from build123d import *

# Parameters (mm, degrees)
F3_DEPTH = 50
F4_DEPTH = 50
F5_DEPTH = 50


with BuildPart() as f3:
    # F0 (on Top) → F3 (new body, symmetric)
    with BuildSketch(Plane.XY):
        with BuildLine():
            Line((-30, 30), (45, 30))
            ThreePointArc((45, 30), (48.535534, 31.464466), (50, 35))
            Line((50, 35), (50, 45))
            ThreePointArc((50, 45), (48.535534, 48.535534), (45, 50))
            Line((45, 50), (-45, 50))
            ThreePointArc((-45, 50), (-48.535534, 48.535534), (-50, 45))
            Line((-50, 45), (-50, -45))
            ThreePointArc((-50, -45), (-48.535534, -48.535534), (-45, -50))
            Line((-45, -50), (45, -50))
            ThreePointArc((45, -50), (48.535534, -48.535534), (50, -45))
            Line((50, -45), (50, 4.584678))
            ThreePointArc((50, 4.584678), (48.535534, 8.120212), (45, 9.584678))
            Line((45, 9.584678), (-16.822587, 9.584678))
            ThreePointArc((-16.822587, 9.584678), (-20.358121, 8.120212), (-21.822587, 4.584678))
            Line((-21.822587, 4.584678), (-21.822587, -15.415322))
            ThreePointArc((-21.822587, -15.415322), (-20.358121, -18.950856), (-16.822587, -20.415322))
            Line((-16.822587, -20.415322), (-13.330647, -20.415322))
            ThreePointArc((-13.330647, -20.415322), (-9.795113, -18.950856), (-8.330647, -15.415322))
            Line((-8.330647, -15.415322), (-8.330647, -5.415322))
            Line((-8.330647, -5.415322), (30, -5.415322))
            Line((30, -5.415322), (30, -30))
            Line((30, -30), (-30, -30))
            Line((-30, -30), (-30, 30))
        make_face()
    extrude(amount=F3_DEPTH, both=True)

    # F1 (on Front) → F4 (intersect, symmetric)
    with BuildSketch(Plane.XZ):
        with BuildLine():
            Line((-33.193547, 7.949598), (-33.193547, 31.362906))
            Line((-33.193547, 31.362906), (45, 31.362906))
            ThreePointArc((45, 31.362906), (48.535534, 32.827372), (50, 36.362906))
            Line((50, 36.362906), (50, 45))
            ThreePointArc((50, 45), (48.535534, 48.535534), (45, 50))
            Line((45, 50), (-45, 50))
            ThreePointArc((-45, 50), (-48.535534, 48.535534), (-50, 45))
            Line((-50, 45), (-50, -45))
            ThreePointArc((-50, -45), (-48.535534, -48.535534), (-45, -50))
            Line((-45, -50), (45, -50))
            ThreePointArc((45, -50), (48.535534, -48.535534), (50, -45))
            Line((50, -45), (50, -37.162689))
            ThreePointArc((50, -37.162689), (48.535534, -33.627155), (45, -32.162689))
            Line((45, -32.162689), (-31.415325, -32.162689))
            Line((-31.415325, -32.162689), (-31.415325, -9.536289))
            Line((-31.415325, -9.536289), (45, -9.536289))
            ThreePointArc((45, -9.536289), (48.535534, -8.071823), (50, -4.536289))
            Line((50, -4.536289), (50, 2.949598))
            ThreePointArc((50, 2.949598), (48.535534, 6.485132), (45, 7.949598))
            Line((45, 7.949598), (-33.193547, 7.949598))
        make_face()
    extrude(amount=F4_DEPTH, both=True, mode=Mode.INTERSECT)

    # F2 (on Right) → F5 (intersect, symmetric)
    with BuildSketch(Plane.YZ):
        with BuildLine():
            ThreePointArc((-45, 50), (-48.535534, 48.535534), (-50, 45))
            Line((-50, 45), (-50, -5))
            ThreePointArc((-50, -5), (-48.535534, -8.535534), (-45, -10))
            Line((-45, -10), (30, -10))
            Line((30, -10), (30, -30))
            Line((30, -30), (-45, -30))
            ThreePointArc((-45, -30), (-48.535534, -31.464466), (-50, -35))
            Line((-50, -35), (-50, -45))
            ThreePointArc((-50, -45), (-48.535534, -48.535534), (-45, -50))
            Line((-45, -50), (45, -50))
            ThreePointArc((45, -50), (48.535534, -48.535534), (50, -45))
            Line((50, -45), (50, 5))
            ThreePointArc((50, 5), (48.535534, 8.535534), (45, 10))
            Line((45, 10), (-30, 10))
            Line((-30, 10), (-30, 30))
            Line((-30, 30), (45, 30))
            ThreePointArc((45, 30), (48.535534, 31.464466), (50, 35))
            Line((50, 35), (50, 45))
            ThreePointArc((50, 45), (48.535534, 48.535534), (45, 50))
            Line((45, 50), (-45, 50))
        make_face()
    extrude(amount=F5_DEPTH, both=True, mode=Mode.INTERSECT)


solid = f3.part
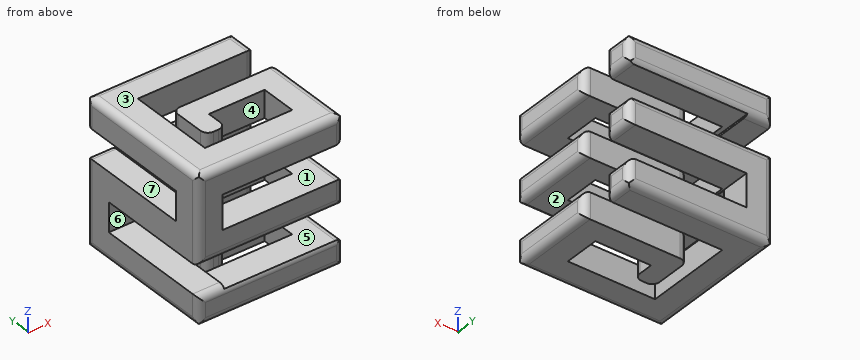
Build history of the part. All positions in model axes, mm. Face numbers are marked on the shaded views. A direction names the side the tool comes from. Give positions to 0.01 mm unless a question says otherwise; leave off trailing zeros. Loops run counter-clockwise (first coordinate to the right, second up) from the corner with the lowest first, then second, coordinate; pieces in that order, holes last. Notation, with made-up numbers: (88.5, 48) - (140.5, 48) arc R22 cw to (140.5, 62) - close; hole circle Ø1 at (79, 13). An arc over 180 degrees is marked (long way). Write item = value, one per line. Start each with the question number.
1) Band-saw the part on B-B on y = 38.5. Give the cut face in (x, z).
2) Band-saw the part on A-A on y = 23.5. Give the cut face in (x, z), plus the area to 3 significant figures.
3) Pull direction Z, two halves, no side cores. Call the marked faces 1, 2, 3 and 4: +Z half, -Z half, draft (parallel to the pull), parting line (faces both ways), or undercut.
4) Tool access for the marked faces 5, 6 and 7: list every direction of +Z, -Z, +X, -X, +Y, -Y with a clear straight run to the whole face (end or side of a thin tool).
5) Probe probe 1 along Z at (x, y) = (-43.5, -21); probe 2 along Z at (x, y) = (-5.5, 9.5); probe 3 along Y at (x, z) = (34.5, 2). List the from-to ranges inside material, lowest first. Write a range as from..to.
6) Band-saw the part on C-C on x = -28. Count the separate pieces of the cut face and the enclosed holes in it, plus the area to 3 significant figures.
7) Band-saw the part on D-D on x = -39. Give the cut face in (y, z), plus the area to 3 significant figures.
Final values:
q1.outline = (-50, -45) arc R5 ccw to (-45, -50) - (45, -50) arc R5 ccw to (50, -45) - (50, -37.16) arc R5 ccw to (45, -32.16) - (-31.42, -32.16) - (-31.42, -9.54) - (45, -9.54) arc R5 ccw to (50, -4.54) - (50, 2.95) arc R5 ccw to (45, 7.95) - (-33.19, 7.95) - (-33.19, 10) - (-50, 10) - close; (-50, 30) - (-33.19, 30) - (-33.19, 31.36) - (45, 31.36) arc R5 ccw to (50, 36.36) - (50, 45) arc R5 ccw to (45, 50) - (-45, 50) arc R5 ccw to (-50, 45) - close
q2.outline = (-50, -45) arc R5 ccw to (-45, -50) - (-30, -50) - (-30, -32.16) - (-31.42, -32.16) - (-31.42, -30) - (-50, -30) - close; (-50, -10) - (-31.42, -10) - (-31.42, -9.54) - (-30, -9.54) - (-30, 7.95) - (-33.19, 7.95) - (-33.19, 10) - (-50, 10) - close; (-50, 30) - (-33.19, 30) - (-33.19, 31.36) - (-30, 31.36) - (-30, 50) - (-45, 50) arc R5 ccw to (-50, 45) - close
q2.area = 1,170 mm²
q3.face_1 = undercut
q3.face_2 = undercut
q3.face_3 = +Z half
q3.face_4 = draft
q4.face_5 = +X, +Y, -Y
q4.face_6 = +X, -X, -Y
q4.face_7 = +X, -X, +Y
q5.probe_1 = -50..-30, -10..10, 30..50
q5.probe_2 = -50..-32.16, -9.54..7.95, 31.36..50
q5.probe_3 = -50..9.58, 30..50
q6.separate_pieces = 6
q6.enclosed_holes = 0
q6.area = 2,130 mm²
q7.outline = (-50, -45) arc R5 ccw to (-45, -50) - (45, -50) arc R5 ccw to (50, -45) - (50, 5) arc R5 ccw to (45, 10) - (-30, 10) - (-30, 30) - (45, 30) arc R5 ccw to (50, 35) - (50, 45) arc R5 ccw to (45, 50) - (-45, 50) arc R5 ccw to (-50, 45) - (-50, -5) arc R5 ccw to (-45, -10) - (30, -10) - (30, -30) - (-45, -30) arc R5 ccw to (-50, -35) - close
q7.area = 6,760 mm²
